```python
from build123d import *

# Parameters (mm, degrees)
F0_R     = 3
F0_R_2   = 13
F1_DEPTH = 12
F2_SIZE  = 10
F3_R     = 2.5
F4_DEPTH = 25
F5_R     = 5.25
F5_R_2   = 3
F6_DEPTH = 6


with BuildPart() as f1:
    # F0 (on Front) → F1 (new body)
    with BuildSketch(Plane.XZ):
        Polygon((0, 145), (0, 0), (80, 0), (80, 220), (-55, 220), (-55, 145), align=None)
        with Locations((6, 20)):
            Circle(F0_R, mode=Mode.SUBTRACT)
        with Locations((6, 80)):
            Circle(F0_R, mode=Mode.SUBTRACT)
        with Locations((74, 20)):
            Circle(F0_R, mode=Mode.SUBTRACT)
        with Locations((74, 80)):
            Circle(F0_R, mode=Mode.SUBTRACT)
        with Locations((-32, 182.5)):
            Circle(F0_R_2, mode=Mode.SUBTRACT)
    extrude(amount=F1_DEPTH)

    # F2
    f2_edges = [f1.edges().sort_by_distance(p)[0] for p in [
        (-55, -6, 220),
        (-55, -6, 145),
    ]]
    chamfer(f2_edges, length=F2_SIZE)

    # F3 (on face) → F4 (cut)
    with BuildSketch(Plane(origin=(-55, 0, 0), x_dir=(0, -1, 0), z_dir=(-1, 0, 0))):
        with Locations((6, 182.5)):
            Circle(F3_R)
    extrude(amount=-F4_DEPTH, mode=Mode.SUBTRACT)

    # F5 (on face) → F6 (cut)
    with BuildSketch(Plane(origin=(0, 0, 0), x_dir=(-1, 0, 0), z_dir=(0, 1, 0))):
        with Locations((-74, 80)):
            Circle(F5_R)
        with Locations((-74, 80)):
            Circle(F5_R_2, mode=Mode.SUBTRACT)
        with Locations((-6, 80)):
            Circle(F5_R)
        with Locations((-6, 80)):
            Circle(F5_R_2, mode=Mode.SUBTRACT)
        with Locations((-6, 20)):
            Circle(F5_R)
        with Locations((-6, 20)):
            Circle(F5_R_2, mode=Mode.SUBTRACT)
        with Locations((-74, 20)):
            Circle(F5_R)
        with Locations((-74, 20)):
            Circle(F5_R_2, mode=Mode.SUBTRACT)
    extrude(amount=-F6_DEPTH, mode=Mode.SUBTRACT)


solid = f1.part
```
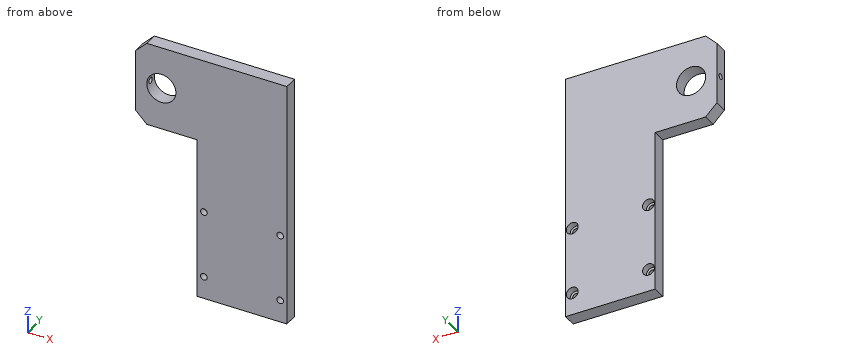
Source: CAD feature listing. Evaluate the final solid. Frame: model axes, mm. Give positions to 0.01 mm unless a question says otherwise; leave off trailing zeros. Order: outer loops, then holes, each group sorted by start corner. A loop starts at its lowest first (then second) coordinate and runs counter-clockwise, first axis right, second up.
(1) Section query A-A (x = 74). Return the cut outline in (y, z).
(2) Contact query for a flat-ended pin moving along its axis: P1, Ø9.5, axis at x = 74, z = 80, coming from the +Y side. Output: stop coordinate, or through.
(3) Section query D-D (z = 80). Return the cut outline in (x, y).
(4) Section query B-B (z = 182.5). Return the cut outline in (x, y), plus the area to 3 significant figures.
(5) Material intervals for line 1 along X through (y, z) = (-8.4, 20); line 2 along Z through (x, y) = (74, -3.45); line 3 along Z through (x, y) = (6, -9.25), sorted ascending.
(6) Section query C-C (x = -32). Return the cut outline in (y, z).
Outcome:
1. outline: (-12, 0) - (0, 0) - (0, 14.75) - (-6, 14.75) - (-6, 17) - (-12, 17) - close; (-12, 23) - (-6, 23) - (-6, 25.25) - (0, 25.25) - (0, 74.75) - (-6, 74.75) - (-6, 77) - (-12, 77) - close; (-12, 83) - (-6, 83) - (-6, 85.25) - (0, 85.25) - (0, 220) - (-12, 220) - close
2. P1: stops at y = -6
3. outline: (0, -12) - (3, -12) - (3, -6) - (0.75, -6) - (0.75, 0) - (0, 0) - close; (9, -12) - (71, -12) - (71, -6) - (68.75, -6) - (68.75, 0) - (11.25, 0) - (11.25, -6) - (9, -6) - close; (77, -12) - (80, -12) - (80, 0) - (79.25, 0) - (79.25, -6) - (77, -6) - close
4. outline: (-55, -12) - (-45, -12) - (-45, -8.5) - (-55, -8.5) - close; (-55, -3.5) - (-45, -3.5) - (-45, 0) - (-55, 0) - close; (-19, -12) - (80, -12) - (80, 0) - (-19, 0) - close
4. area: 1,260 mm2
5. line 1: x = 0 to 3, 9 to 71, 77 to 80
5. line 2: z = 0 to 14.75, 25.25 to 74.75, 85.25 to 220
5. line 3: z = 0 to 17, 23 to 77, 83 to 220
6. outline: (-12, 145) - (0, 145) - (0, 169.5) - (-12, 169.5) - close; (-12, 195.5) - (0, 195.5) - (0, 220) - (-12, 220) - close
